Model file for the job. Use its own axes, mm. A direction names the side the tool comes from. Coordinates: 2 decimals unless noted, no trailing zeros. Order: outer loops, then holes, each group sorted by start corner. A loop starts at its lowest first (then second) coordinate and runs counter-clockwise, first axis right, second up.
from build123d import *

# Parameters (mm, degrees)
SKETCH_1_W               = 65.34
SKETCH_1_H               = 61.875
EXTRUDE_1_DEPTH          = 5.1
CUT_EXTRUDE_1_DEPTH      = 0.5
SKETCH_2_3_W             = 1.1
SKETCH_2_3_H             = 24.9
CUT_EXTRUDE_2_DEPTH      = 0.5
SKETCH_3_OUTSIDE_W       = 85.366
SKETCH_3_OUTSIDE_H       = 81.901
SKETCH_3_OUTSIDE_W_2     = 65.34
SKETCH_3_OUTSIDE_H_2     = 61.875
SKETCH_3_OUTSIDE_W_3     = 64.34
SKETCH_3_OUTSIDE_H_3     = 60.88
CUT_EXTRUDE_4_DEPTH      = 5
CUT_EXTRUDE_6_DEPTH      = 91.13235393
CUT_EXTRUDE_6_DEPTH_BACK = 91.13235393
CUT_EXTRUDE_7_DEPTH      = 91.13235393
CUT_EXTRUDE_7_DEPTH_BACK = 0.6
CUT_EXTRUDE_START        = -0.5
CUT_EXTRUDE_8_OUTLINE_W  = 2
CUT_EXTRUDE_8_OUTLINE_H  = 2.5
CUT_EXTRUDE_8_DEPTH      = 0.5


# Read off the part's stored shape, not the designer's step: 切除-拉伸8
with BuildPart() as part:
    # 草图1 → 凸台-拉伸1 (new body)
    with BuildSketch(Plane.XY):
        with Locations((32.67, 30.9375)):
            Rectangle(SKETCH_1_W, SKETCH_1_H)
    extrude(amount=EXTRUDE_1_DEPTH)

    # 草图2 → 切除-拉伸1 (cut)
    with BuildSketch(Plane(origin=(65.34, 0, 0), x_dir=(0, 0, -1), z_dir=(1, 0, 0))):
        Polygon((0, 28.5), (0, 60.075), (-1.1, 60.075), (-1.1, 51.6), (-4.1, 51.6), (-4.1, 46.6), (-1.1, 46.6), (-1.1, 28.5), align=None)
    extrude(amount=-CUT_EXTRUDE_1_DEPTH, mode=Mode.SUBTRACT)

    # 草图2<3> → 切除-拉伸2 (cut)
    with BuildSketch(Plane(origin=(65.34, 0, 0), x_dir=(0, 0, -1), z_dir=(1, 0, 0))):
        with Locations((-0.55, 14.25)):
            Rectangle(SKETCH_2_3_W, SKETCH_2_3_H)
    extrude(amount=-CUT_EXTRUDE_2_DEPTH, mode=Mode.SUBTRACT)

    # 草图3 outside → 切除-拉伸4 (cut)
    # profile 1 of 2: a face of its own
    with BuildSketch(Plane(origin=(0, 0, 0), x_dir=(-1, 0, 0), z_dir=(0, 0, -1))):
        with Locations((-32.67, 30.9375)):
            Rectangle(SKETCH_3_OUTSIDE_W, SKETCH_3_OUTSIDE_H)
        with Locations((-32.67, 30.9375)):
            Rectangle(SKETCH_3_OUTSIDE_W_2, SKETCH_3_OUTSIDE_H_2, mode=Mode.SUBTRACT)
    # profile 2 of 2: a face of its own
    with BuildSketch(Plane(origin=(0, 0, 0), x_dir=(-1, 0, 0), z_dir=(0, 0, -1))):
        with Locations((-32.67, 30.94)):
            Rectangle(SKETCH_3_OUTSIDE_W_3, SKETCH_3_OUTSIDE_H_3)
    extrude(amount=-CUT_EXTRUDE_4_DEPTH, mode=Mode.SUBTRACT)

    # 草图6 → 切除-拉伸6 (cut, two sides: drawn at the far end of the back side and taken through both)
    with BuildSketch(Plane(origin=(0, 0, 0), x_dir=(1, 0, 0), z_dir=(0, 1, 0)).offset(-CUT_EXTRUDE_6_DEPTH_BACK)):
        Polygon((-141.077467171, 0), (0, 0), (1.8, 0), (1.8, -1.1), (21.875, -1.1), (21.875, 0), (23.675, 0), (23.675, -1.1), (43.675, -1.1), (43.675, 0), (45.475, 0), (45.475, -1.1), (63.54, -1.1), (63.54, 0), (65.34, 0), (206.417467171, 0), (206.417467171, 282.154934342), (-141.077467171, 282.154934342), align=None)
    extrude(amount=CUT_EXTRUDE_6_DEPTH + CUT_EXTRUDE_6_DEPTH_BACK, mode=Mode.SUBTRACT)

    # 草图13 → 切除-拉伸7 (cut, two sides: drawn at the far end of the back side and taken through both)
    with BuildSketch(Plane.ZY.offset(-CUT_EXTRUDE_7_DEPTH_BACK)):
        Polygon((1.1, 60.075), (0, 60.075), (0, 1.8), (1.1, 1.8), (1.1, 10.6), (4.1, 10.6), (4.1, 35.075), (1.1, 35.075), align=None)
    extrude(amount=CUT_EXTRUDE_7_DEPTH + CUT_EXTRUDE_7_DEPTH_BACK, mode=Mode.SUBTRACT)

    # 切除-拉伸8 outline → 切除-拉伸8 (cut)
    with BuildSketch(Plane(origin=(65.34, 0, 0), x_dir=(0, 0, -1), z_dir=(1, 0, 0)).offset(CUT_EXTRUDE_START)):
        with Locations((-2.1, 32.15)):
            Rectangle(CUT_EXTRUDE_8_OUTLINE_W, CUT_EXTRUDE_8_OUTLINE_H)
        with Locations((-2.1, 37.65)):
            Rectangle(CUT_EXTRUDE_8_OUTLINE_W, CUT_EXTRUDE_8_OUTLINE_H)
    extrude(amount=CUT_EXTRUDE_8_DEPTH, mode=Mode.SUBTRACT)


solid = part.part
Q1. Cut at B-B, the plane x = 33.5. List the corners of the cut face in (y, z) (3 decimals), plus the area to 3 significant figures.
Established:
outline: (0, 1.1) - (0.5, 1.1) - (0.5, 5) - (61.38, 5) - (61.38, 1.1) - (61.875, 1.1) - (61.875, 5.1) - (0, 5.1) - close
area: 10.1 mm2
Q2. Mould opens along Y. For faces 3 (the face through (0.5, 30.5, 4.7)), 4 (the face through (32, 61.875, 3)), 5 (the face through (65.34, 30.5, 3.1)) say: pulls with the +Y half, pulls with the -Y half, needs draft (parallel to the pull), parting line crosses it, or undercut.
Established:
face 3: undercut
face 4: pulls with the +Y half
face 5: needs draft
Q3. Drop flat-ended pins along their axis: P1, Ø3, axis at x = 10.5, y = 40, coming from the -Z side; P2, Ø1.5, axis at y = 34, z = 3, coming from the -X side; P3, Ø0.5, axis at x = 29, y = 61.5, coming from the -Z side. Give the stop position or say it passes through.
Established:
P1: stops at z = 5
P2: stops at x = 64.84
P3: stops at z = 1.1
Q4. Probe line 1 (Y direction, x = 18, z = 4.3) (3 decimals); line 2 (X direction, y = 20, z = 4.95); line 3 (X direction, y = 25.5, z = 2.9). List the from-to ranges inside material, lowest first.
Established:
line 1: y = 0 to 0.5, 61.38 to 61.875
line 2: x = 0 to 0.5, 64.84 to 65.34
line 3: x = 64.84 to 65.34
Q5. Cut at A-A, the plane y = 55.5. List the corners of the cut face in (x, z), plus the area to 3 significant figures.
Established:
outline: (0, 1.1) - (0.5, 1.1) - (0.5, 5) - (64.84, 5) - (64.84, 1.1) - (65.34, 1.1) - (65.34, 5.1) - (0, 5.1) - close
area: 10.4 mm2
Q6. Which spindle directions (+Z, -Z, +X, -X, +Y, -Y) get a long thin tool onto all of the face, cutting with end or side? Do faces 1 (the face through (32, 0, 3)), 2 (the face through (33, 0.5, 3)). Say none if no direction does.
Established:
face 1: +Z, -Z, +X, -X, -Y
face 2: -Z
